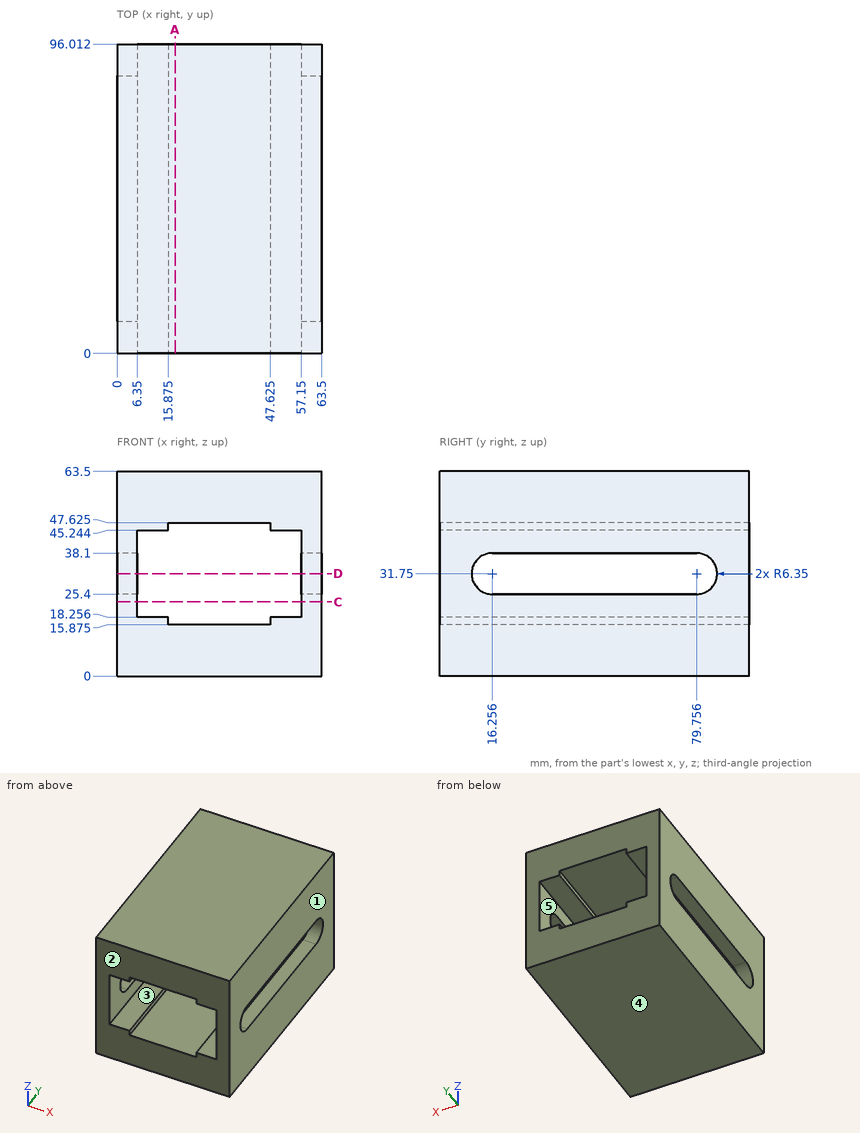
The figure shows three views and two pictorial views of one solid part (mm, origin at its lowest corner). Answer the questions. A direction names the side the tool comes from. Coordinates: 2 decimals unless noted, no trailing zeros. Loops run counter-clockwise (first coordinate to the right, second up) from the corner with the lowest first, then second, coordinate; pieces in that order, holes last. Notation, with made-up numbers: (79, -21.75) -> (119, -21.75) arc R15 cw to (119, -13.75) -> close; hole circle Ø5 at (10, 63). An arc over 180 degrees is marked (long way). Return JSON: item names as keys, results as strings. Group by question number.
(1) A cutting plane is placed at C-C on z = 23. Write down the section's boundary in (x, y), and give its area (3 significant figures).
(2) Which of the six approach directions +Z, -Z, +X, -X, +Y, -Y give full straight-line access (tool end or side, diameter ignored) to the marked faces 4 and 5?
(3) Given pin 1 Ø3 at (y, z) = (26.5, 28) entering from -X, flat-ended and moving along its own axis, determine where the tip first touches the part or whether it passes through.
(4) Determine the mould class of the marked faces 1, 2 and 3 for opening direction X: released by +X, released by -X, zero draft, split by the parting line, or undercut.
(5) A cutting plane is placed at D-D on z = 31.75. Write down the section's boundary in (x, y).
(6) Find the intervals of material crossed by probe 1 along Z at (x, y) = (27, 22) (1 decimal); probe 2 along Z at (x, y) = (13, 10); probe 3 along X at (y, z) = (83, 41), in increasing order. Write a range as from..to.
(7) A cutting plane is placed at A-A on x = 18. Write down the section's boundary in (y, z) (1 decimal).
The answers:
{
 "1": {"outline": "(0, 0) -> (6.35, 0) -> (6.35, 96.01) -> (0, 96.01) -> close; (57.15, 0) -> (63.5, 0) -> (63.5, 96.01) -> (57.15, 96.01) -> close", "area": "1,220 mm^2"},
 "2": {"face 4": "-Z, +X, -X, +Y, -Y", "face 5": "+Y, -Y"},
 "3": {"pin 1": "passes through"},
 "4": {"face 1": "released by +X", "face 2": "zero draft", "face 3": "undercut"},
 "5": {"outline": "(0, 0) -> (6.35, 0) -> (6.35, 9.91) -> (0, 9.91) -> close; (0, 86.11) -> (6.35, 86.11) -> (6.35, 96.01) -> (0, 96.01) -> close; (57.15, 0) -> (63.5, 0) -> (63.5, 9.91) -> (57.15, 9.91) -> close; (57.15, 86.11) -> (63.5, 86.11) -> (63.5, 96.01) -> (57.15, 96.01) -> close"},
 "6": {"probe 1": "z = 0..15.9, 47.6..63.5", "probe 2": "z = 0..18.26, 45.24..63.5", "probe 3": "x = 0..6.35, 57.15..63.5"},
 "7": {"outline": "(0, 0) -> (96, 0) -> (96, 15.9) -> (0, 15.9) -> close; (0, 47.6) -> (96, 47.6) -> (96, 63.5) -> (0, 63.5) -> close"}
}
